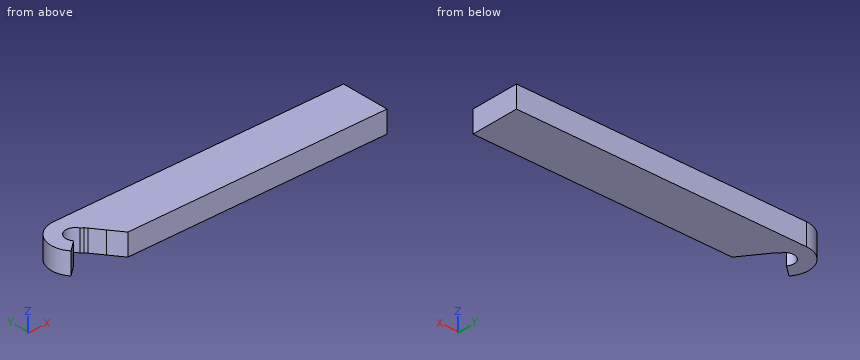
from build123d import *

# Parameters (mm, degrees)
F1_DEPTH    = 3
F2_T4_DEPTH = 7.0269593276


# Not quite as in the source:
# - a fillet or chamfer that OpenCascade refuses, or shapes differently, is made with other operations: its cross-section is extruded or revolved along the edge and cut away or added


with BuildPart() as f1:
    # F0 (on Top) → F1 (new body)
    with BuildSketch(Plane.XY):
        with BuildLine():
            ThreePointArc((-40.9958577761, -0.8356238926), (-40.4446261863, 1.221600407), (-38.7, 0))
            Line((-38.7, 0), (-38.2265411317, 0))
            Line((-38.2265411317, 0), (-36.7, 0))
            ThreePointArc((-36.7, 0), (-36.7956166893, -0.7886238635), (-37.076925817, -1.5315473615))
            Line((-37.076925817, -1.5315473615), (-35.7494838536, -3.3))
            Line((-35.7494838536, -3.3), (0, -3.3))
            Line((0, -3.3), (0, 0))
            Line((0, 0), (0, 3.3))
            Line((0, 3.3), (-40, 3.3))
            ThreePointArc((-40, 3.3), (-42.9908156972, 1.3946402637), (-42.5279466623, -2.121199112))
            Line((-42.5279466623, -2.121199112), (-40.9958577761, -0.8356238926))
        make_face()
        with BuildLine():
            Line((-36.7, 0), (-38.2265411317, 0))
            Line((-38.2265411317, 0), (-37.076925817, -1.5315473615))
            ThreePointArc((-37.076925817, -1.5315473615), (-36.7956166893, -0.7886238635), (-36.7, 0))
        make_face()
    extrude(amount=F1_DEPTH)

    # F2: chamfer of 1 on 1 edges, made by hand


with BuildPart() as f2_tool2:
    # F2_s3 → F2_t4 (new body)
    with BuildSketch(Plane.XY.offset(-2.0134796638)):
        with BuildLine():
            Line((-38.8293039248, 0.5652173913), (-37.9287684823, 0))
            Line((-37.9287684823, 0), (-38.7, 0))
            ThreePointArc((-38.7, 0), (-38.7360904804, 0.3041919232), (-38.8293039248, 0.5652173913))
        make_face()
    extrude(amount=F2_T4_DEPTH)

    split(bisect_by=Plane(origin=(-24.4503471764, -18.3530031596, 0), x_dir=(0, 0, 1), z_dir=(-0.7997606156, -0.6003190466, 0)), keep=Keep.TOP)


with BuildPart() as f1_1:
    add(f1.part)

    # F2_t1: cut F2_tool2
    add(f2_tool2.part, mode=Mode.SUBTRACT)


solid = f1_1.part
Verification items for the finished model (mm, model axes). Coordinates: 2 decimals unless noted, no trailing zeros. Order: outer loops, then holes, each group sorted by start corner. A loop starts at its lowest first (then second) coordinate and runs counter-clockwise, first axis right, second up. Notation, with made-up numbers: M 62,26.5 L 101,26.5 A18 ccw 101,35.5 Z; hole C 73,64.25 d8. An arc over 180 degrees is marked long. One line per item, written item: value. Start each with the question number.
Item 1: Thickness scan on probe 1 along X at (y, z) = (0, 2.1); probe 2 along Y at (x, z) = (-40, 1.5); probe 3 along X at (y, z) = (2.25, 0.95). Record the ranges inside material, lowest first.
Item 2: Sectioned sample at C-C on y = -2.5. Record the cut outline in (x, z), then the cut area to 3 significant figures.
Item 3: Sectioned sample at B-B on y = 2. Record the cut outline in (x, z), then the cut area to 3 significant figures.
Item 4: Depth check by flat-ended pin: P1, Ø1.5, axis at y = -1.5, z = 1, coming from the -X side; P2, Ø1, axis at x = -33.5, y = -2, coming from the -Z side; P3, Ø1.5, axis at y = -1, z = 2.5, coming from the -X side. Enter the tip coordinate at first touch or a pass-through.
Item 5: Sectioned sample at A-A on z = 2.35. Record the cut outline in (x, y), then the cut area to 3 significant figures.
Calculated:
1. probe 1: -43.3 to -41.3, -38.23 to 0
1. probe 2: 1.3 to 3.3
1. probe 3: -42.41 to 0
2. outline: M -36.35,0 L 0,0 L 0,3 L -36.35,3 Z
2. area: 109 mm^2
3. outline: M -42.62,0 L 0,0 L 0,3 L -42.62,3 Z
3. area: 128 mm^2
4. P1: x = -43.21
4. P2: z = 0
4. P3: x = -43.29
5. outline: M -42.53,-2.12 L -41,-0.84 A1.3 cw long -38.83,0.57 L -38.49,0.35 L -35.75,-3.3 L 0,-3.3 L 0,3.3 L -40,3.3 A3.3 ccw Z
5. area: 263 mm^2
